Geometry: final body of the model. Coordinates: model frame, mm. A direction names the side the tool comes from. Round coordinates to 2 decimals unless told otherwise and drop trailing zeros. Write each loop counter-clockwise with the first axis right and the second up, starting at its lowest first coordinate (ties: lowest second). Pieces come first, ordered by that corner, then holes.
from build123d import *

# Parameters (mm, degrees)
SKETCH11_W          = 38.1
SKETCH11_H          = 38.1
SKETCH12_W          = 38.1
SKETCH12_H          = 38.1
BOSS_EXTRUDE5_DEPTH = 12.7
BOSS_EXTRUDE5_TAPER = 20
BOSS_EXTRUDE6_DEPTH = 38.1
SKETCH14_R          = 7.62
CUT_EXTRUDE2_DEPTH  = 38.1
SKETCH15_R          = 12.065
CUT_EXTRUDE3_DEPTH  = 12.7
CUT_EXTRUDE4_DEPTH  = 38.1


with BuildPart() as part:
    # Sweep1: sweep along a path in Sketch10
    with BuildLine(Plane(origin=(0, 0, 0), x_dir=(0, 0, -1), z_dir=(1, 0, 0))) as sweep1_path:
        Line((0, 96.393), (0, 25.4))
        Line((0, 25.4), (-25.4, 0))
    # Sketch11 → Sweep1 (sweep)
    with BuildSketch(Plane(origin=(0, 96.393, 0), x_dir=(1, 0, 0), z_dir=(0, 1, 0))):
        Rectangle(SKETCH11_W, SKETCH11_H)
    sweep(path=sweep1_path.line, transition=Transition.RIGHT)

    # Sketch12 → Boss-Extrude5 (add)
    with BuildSketch(Plane(origin=(0, -12.7, 12.7), x_dir=(1, 0, 0), z_dir=(0, -0.7071067811865461, 0.7071067811865489))):
        with Locations((0, 17.960512242)):
            Rectangle(SKETCH12_W, SKETCH12_H)
    extrude(amount=BOSS_EXTRUDE5_DEPTH, taper=BOSS_EXTRUDE5_TAPER)

    # Sketch13 → Boss-Extrude6 (add)
    with BuildSketch(Plane(origin=(0, 0, -19.05), x_dir=(-1, 0, 0), z_dir=(0, 0, -1))):
        with BuildLine():
            Line((-19.05, 96.393), (19.05, 96.393))
            ThreePointArc((19.05, 96.393), (0, 115.443), (-19.05, 96.393))
        make_face()
    extrude(amount=-BOSS_EXTRUDE6_DEPTH)

    # Sketch14 → Cut-Extrude2 (cut)
    with BuildSketch(Plane.XY.offset(19.05)):
        with Locations((0, 96.393)):
            Circle(SKETCH14_R)
    extrude(amount=-CUT_EXTRUDE2_DEPTH, mode=Mode.SUBTRACT)

    # Sketch15 → Cut-Extrude3 (cut)
    with BuildSketch(Plane(origin=(0, -21.680256121, 21.680256121), x_dir=(1, 0, 0), z_dir=(0, -0.7071067811865461, 0.7071067811865489))):
        with Locations(Location((0, 17.960512242, 0), (0, 0, 270))):
            Circle(SKETCH15_R)
    extrude(amount=-CUT_EXTRUDE3_DEPTH, mode=Mode.SUBTRACT)

    # Sketch16 → Cut-Extrude4 (cut)
    with BuildSketch(Plane.ZY.offset(19.05)):
        Polygon((-10.345169525, 82.99999799), (10.345169525, 82.99999799), (0, 67.376680748), align=None)
        Polygon((10.345169525, 39.968335079), (0, 55.591652321), (-10.345169525, 39.968335079), align=None)
    extrude(amount=-CUT_EXTRUDE4_DEPTH, mode=Mode.SUBTRACT)


solid = part.part
1) Section B-B on x = 0. Output: boundary loops of the cut face in (y, z).
2) Section C-C on y = 65.5. Output: boundary loops of the cut face in (x, z), plus the area to 3 significant figures.
3) Line query: probe 1 along Y at (x, z) = (0, 0); probe 2 along Y at (x, z) = (9, -8); probe 3 along Y at (x, z) = (0, -4.5). Output: solid intervals per line, ascending.
4) First-contact query: P1, Ø12, axis at x = 11, y = 89, coming from the +Z side; P2, Ø16.5, axis at x = -2, z = 5, coming from the +Y side; P3, Ø6, axis at x = 5, z = 1.5, coming from the -Y side; P4, Ø6, axis at x = -14, z = 27, coming from the -Y side. Flat tips, straight axial feed; report the tip coordinate or a pass-through.
5) Draft query along Z for faces 3 (the flat face through (0.2, 0.1, 25.5)), 4 (the cylindrical face through (-0.42, 115.44, -0.27)), 5 (the flat face through (-0.27, 75.08, -5.1)), 6 (the flat face through (16.77, -4.24, 30.02)). Return one class per face: pulls with the +Z half, pulls with the -Z half, needs draft (parallel to the pull), parting line crosses it, or undercut.
6) Section A-A on z = 3.5. Output: boundary loops of the cut face in (x, y), plus the area to 3 significant figures.
7) Reachability of faces 1 (the flat face through (-19.05, 53, 3)), 2 (the flat face through (-0.267, 47.671, 5.245)) from +Z, -Z, +X, -X, +Y, -Y: full face, straight path, thin tool, end or side. Return the list, or none.
8) Section D-D on z = -8.5. Output: boundary loops of the cut face in (x, y), plus the area to 3 significant figures.
Filled in:
1. outline: (-19.18, 24.18) - (-13.47, 11.93) - (17.51, -19.05) - (88.77, -19.05) - (88.77, 19.05) - (33.29, 19.05) - (13.47, 38.87) - (1.22, 44.58) - (-0.45, 42.91) - (8.53, 33.93) - (-8.53, 16.87) - (-17.51, 25.85) - close; (104.01, -19.05) - (115.44, -19.05) - (115.44, 19.05) - (104.01, 19.05) - close; hole (39.97, -10.35) - (55.59, 0) - (39.97, 10.35) - close; hole (67.38, 0) - (83, -10.35) - (83, 10.35) - close
2. outline: (-19.05, -19.05) - (19.05, -19.05) - (19.05, 19.05) - (-19.05, 19.05) - close
2. area: 1,450 mm2
3. probe 1: y = -1.54 to 39.97, 55.59 to 67.38, 83 to 88.77, 104.01 to 115.44
3. probe 2: y = 6.46 to 39.97, 43.51 to 79.46, 83 to 113.18
3. probe 3: y = 2.96 to 39.97, 48.8 to 74.17, 83 to 88.77, 104.01 to 115.44
4. P1: stops at z = 19.05
4. P2: stops at y = 115.44
4. P3: stops at y = -6.04
4. P4: stops at y = -19.18
5. face 3: undercut
5. face 4: needs draft
5. face 5: undercut
5. face 6: pulls with the +Z half
6. outline: (-19.05, -5.04) - (19.05, -5.04) - (19.05, 39.97) - (-19.05, 39.97) - close; (-19.05, 50.31) - (19.05, 50.31) - (19.05, 72.66) - (-19.05, 72.66) - close; (-19.05, 83) - (19.05, 83) - (19.05, 96.39) arc R19.05 ccw to (-19.05, 96.39) - close; hole circle Ø15.24 at (0, 96.39)
6. area: 3,460 mm2
7. face 1: +Z, -Z, -X, +Y, -Y
7. face 2: +X, -X
8. outline: (-19.05, 6.96) - (19.05, 6.96) - (19.05, 39.97) - (-19.05, 39.97) - close; (-19.05, 42.75) - (19.05, 42.75) - (19.05, 80.21) - (-19.05, 80.21) - close; (-19.05, 83) - (19.05, 83) - (19.05, 96.39) arc R19.05 ccw to (-19.05, 96.39) - close; hole circle Ø15.24 at (0, 96.39)
8. area: 3,580 mm2
